Source: CAD feature listing. Evaluate the final solid. Frame: model axes, mm. Face numbers are marked on the shaded views. A direction names the side the tool comes from. Round coordinates to 2 decimals unless told otherwise and drop trailing zeros. Write each loop counter-clockwise with the first axis right and the second up, starting at its lowest first coordinate (ties: lowest second). Pieces come first, ordered by that corner, then holes. Notation, with made-up numbers: (33.25, -38.5) - (41.25, -38.5) arc R14 ccw to (41.25, -32.5) - close; hole circle Ø8 at (9, -22.75). An arc over 180 degrees is marked (long way). Write item = value, one per line. Start each with the question number.
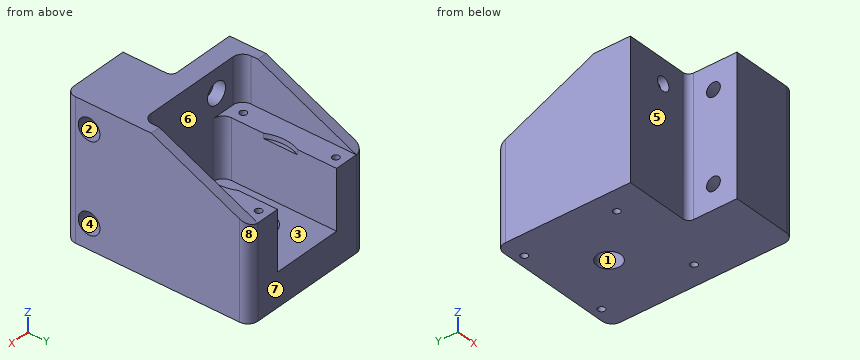
```python
from build123d import *

# Parameters (mm, degrees)
SKETCH1_R                                       = 1.75
SKETCH1_R_2                                     = 6
BOSS_EXTRUDE1_DEPTH                             = 70
SKETCH2_W                                       = 60
SKETCH2_H                                       = 58.5
CUT_EXTRUDE2_DEPTH                              = 23
CUT_EXTRUDE3_DEPTH                              = 53
CUT_EXTRUDE5_START                              = -23
CUT_EXTRUDE5_DEPTH                              = 2.5
SKETCH5_R                                       = 11.1
CUT_EXTRUDE4_DEPTH                              = 7
CHAMFER1_SIZE                                   = 50
CHAMFER1_SIZE2                                  = 23
FILLET1_R                                       = 5
FILLET2_R                                       = 5
CBORE_FOR_M6_SOCKET_HEAD_CAP_SCREW1_D           = 7
CBORE_FOR_M6_SOCKET_HEAD_CAP_SCREW1_CBORE_D     = 11
CBORE_FOR_M6_SOCKET_HEAD_CAP_SCREW1_CBORE_DEPTH = 6
CBORE_FOR_M6_SOCKET_HEAD_CAP_SCREW2_D           = 7
CBORE_FOR_M6_SOCKET_HEAD_CAP_SCREW2_CBORE_D     = 11
CBORE_FOR_M6_SOCKET_HEAD_CAP_SCREW2_CBORE_DEPTH = 15
CHAMFER2_SIZE                                   = 1


with BuildPart() as part:
    # Sketch1 → Boss-Extrude1 (new body)
    with BuildSketch(Plane.XY):
        with BuildLine():
            Line((35, 28.5), (-35, 28.5))
            Line((-35, 28.5), (-35, -25))
            Line((-35, -25), (-35, -40))
            Line((-35, -40), (-3, -40))
            ThreePointArc((-3, -40), (-0.878679656, -40.878679656), (0, -43))
            Line((0, -43), (0, -65))
            Line((0, -65), (35, -65))
            Line((35, -65), (35, -25))
            Line((35, -25), (35, 28.5))
        make_face()
        with Locations((-23.5, -23.5)):
            Circle(SKETCH1_R, mode=Mode.SUBTRACT)
        with Locations((23.5, -23.5)):
            Circle(SKETCH1_R, mode=Mode.SUBTRACT)
        Circle(SKETCH1_R_2, mode=Mode.SUBTRACT)
        with Locations((-23.5, 23.5)):
            Circle(SKETCH1_R, mode=Mode.SUBTRACT)
        with Locations((23.5, 23.5)):
            Circle(SKETCH1_R, mode=Mode.SUBTRACT)
    extrude(amount=-BOSS_EXTRUDE1_DEPTH)

    # Sketch2 → Cut-Extrude2 (cut)
    with BuildSketch(Plane.XY):
        with Locations((0, -0.75)):
            Rectangle(SKETCH2_W, SKETCH2_H)
    extrude(amount=-CUT_EXTRUDE2_DEPTH, mode=Mode.SUBTRACT)

    # Sketch6 → Cut-Extrude3 (cut)
    with BuildSketch(Plane.XY):
        Polygon((-18, -8.717797887), (-18, -30), (18, -30), (18, -8.717797887), (18, 8.717797887), (18, 28.5), (-18, 28.5), (-18, 8.717797887), align=None)
    extrude(amount=-CUT_EXTRUDE3_DEPTH, mode=Mode.SUBTRACT)

    # Sketch6<4> → Cut-Extrude5 (cut)
    with BuildSketch(Plane.XY.offset(CUT_EXTRUDE5_START)):
        with BuildLine():
            Line((-18, 8.717797887), (-18, -8.717797887))
            ThreePointArc((-18, -8.717797887), (-20, 0), (-18, 8.717797887))
        make_face()
        with BuildLine():
            Line((18, 8.717797887), (18, -8.717797887))
            ThreePointArc((18, -8.717797887), (20, 0), (18, 8.717797887))
        make_face()
    extrude(amount=-CUT_EXTRUDE5_DEPTH, mode=Mode.SUBTRACT)

    # Sketch5 → Cut-Extrude4 (cut)
    with BuildSketch(Plane.XY.offset(-53)):
        Circle(SKETCH5_R)
    extrude(amount=-CUT_EXTRUDE4_DEPTH, mode=Mode.SUBTRACT)

    # Chamfer1
    chamfer1_edges = [part.edges().sort_by_distance(p)[0] for p in [
        (32.5, 28.5, 0),
        (-32.5, 28.5, 0),
    ]]
    chamfer1_side = [part.faces().sort_by_distance(p)[0] for p in [
        (7.08218847, -32.820097977, 0),
    ]]
    chamfer(chamfer1_edges, length=CHAMFER1_SIZE, length2=CHAMFER1_SIZE2, reference=chamfer1_side[0])

    # Fillet1
    fillet1_edges = [part.edges().sort_by_distance(p)[0] for p in [
        (35, -65, -35),
        (35, 28.5, -46.5),
        (-35, 28.5, -46.5),
    ]]
    fillet(fillet1_edges, radius=FILLET1_R)

    # Fillet2
    fillet2_edges = [part.edges().sort_by_distance(p)[0] for p in [
        (30, -30, -11.5),
        (-30, -30, -11.5),
        (18, -30, -38),
        (-18, -30, -38),
    ]]
    fillet(fillet2_edges, radius=FILLET2_R)

    # CBORE for M6 Socket Head Cap Screw1 (through all)
    with Locations(Plane(origin=(-15, -30, -12), x_dir=(1, 0, 0), z_dir=(0, 1, 0))):
        with Locations((0, 0)):
            CounterBoreHole(CBORE_FOR_M6_SOCKET_HEAD_CAP_SCREW1_D / 2, CBORE_FOR_M6_SOCKET_HEAD_CAP_SCREW1_CBORE_D / 2, CBORE_FOR_M6_SOCKET_HEAD_CAP_SCREW1_CBORE_DEPTH)

    # CBORE for M6 Socket Head Cap Screw2 (through all)
    with Locations(Plane(origin=(35, 0, 0), x_dir=(0, 0, -1), z_dir=(1, 0, 0))):
        with Locations((12.5, -53), (57.5, -53)):
            CounterBoreHole(CBORE_FOR_M6_SOCKET_HEAD_CAP_SCREW2_D / 2, CBORE_FOR_M6_SOCKET_HEAD_CAP_SCREW2_CBORE_D / 2, CBORE_FOR_M6_SOCKET_HEAD_CAP_SCREW2_CBORE_DEPTH)

    # Chamfer2
    chamfer2_edges = [part.edges().sort_by_distance(p)[0] for p in [
        (-6, 0, -60),
    ]]
    chamfer(chamfer2_edges, length=CHAMFER2_SIZE)


solid = part.part
```
(1) Contact query for flat-ended pins moving along their axis: P1, Ø2, axis at x = -16, z = -34.5, coming from the -Y side; P2, Ø4, axis at x = -15, z = -12, coming from the +Y side; P3, Ø1, axis at x = -10, z = -30, coming from the +Y side; P4, Ø8, axis at y = -53, z = -12.5, coming from the -X side. Output: stop coordinate, or through.
(2) Pull-direction query (Z, two-part tool) for the marked faces 1, 2 and 3; classes: +Z half, -Z half, draft (parallel to the pull), parting line (faces both ways), or undercut.
(3) Section A-A (x = 23.5). Return the cut outline in (y, z), plus the area to 3 significant figures.
(4) Ray query, L1, parallel to Y at x = -23.5, z = -38.5; L2, parallel to X at y = 1, z = -32.5; L3, parallel to Y at x = 5.75, z = -12.5. Return the intervals inside material, ascending. Write a range as from..to.
(5) Section C-C (x = -23.5). Return the cut outline in (y, z), plus the area to 3 significant figures.
(6) Section B-B (z = -57.5). Return the cut outline in (x, y).
(7) Reachability of the marked faces 4, 5, 6, 7 and 8 from +Z, -Z, +X, -X, +Y, -Y: full face, straight path, thin tool, end or side. Return the list, or none.
(8) Section D-D (y = -28). Return the cut outline in (x, z).
Solution:
q1.P1 = -40
q1.P2 = through
q1.P3 = -30
q1.P4 = 0
q2.face_1 = draft
q2.face_2 = undercut
q2.face_3 = +Z half
q3.outline = (-65, -70) - (-25.25, -70) - (-25.25, -23) - (-30, -23) - (-30, 0) - (-65, 0) - close; (-21.75, -70) - (21.75, -70) - (21.75, -23) - (-21.75, -23) - close; (25.25, -70) - (28.5, -70) - (28.5, -23) - (25.25, -23) - close; hole circle Ø11 at (-53, -57.5); hole circle Ø11 at (-53, -12.5)
q3.area = 4,680 mm^2
q4.L1 = -40..-25.25, -21.75..21.75, 25.25..28.5
q4.L2 = -35..-18, 18..35
q4.L3 = -65..-56.5, -49.5..-30
q5.outline = (-40, -70) - (-25.25, -70) - (-25.25, -23) - (-30, -23) - (-30, 0) - (-40, 0) - close; (-21.75, -70) - (21.75, -70) - (21.75, -23) - (-21.75, -23) - close; (25.25, -70) - (28.5, -70) - (28.5, -23) - (25.25, -23) - close
q5.area = 3,120 mm^2
q6.outline = (-35, -40) - (-3, -40) arc R3 cw to (0, -43) - (0, -49.5) - (20, -49.5) - (20, -47.5) - (35, -47.5) - (35, 23.5) arc R5 ccw to (30, 28.5) - (-30, 28.5) arc R5 ccw to (-35, 23.5) - close; (0, -65) - (30, -65) arc R5 ccw to (35, -60) - (35, -58.5) - (20, -58.5) - (20, -56.5) - (0, -56.5) - close; hole circle Ø3.5 at (-23.5, -23.5); hole circle Ø3.5 at (-23.5, 23.5); hole circle Ø22.2 at (0, 0); hole circle Ø3.5 at (23.5, -23.5); hole circle Ø3.5 at (23.5, 23.5)
q7.face_4 = +X
q7.face_5 = +Z, -Z, -X, -Y
q7.face_6 = +Z, +Y
q7.face_7 = +Z, -Z, +X, -X, +Y
q7.face_8 = +Z, -Z, +X, +Y
q8.outline = (-35, -70) - (35, -70) - (35, 0) - (29, 0) - (29, -23) - (17, -23) - (17, -53) - (-17, -53) - (-17, -23) - (-29, -23) - (-29, 0) - (-35, 0) - close
